For this review, take the finished solid that the model builds, in its own axes (mm). A direction names the side the tool comes from. Round coordinates to 2 decimals unless told otherwise and drop trailing zeros. Order: outer loops, then holes, each group sorted by start corner. A loop starts at its lowest first (then second) coordinate and runs counter-clockwise, first axis right, second up. Notation, with made-up numbers: (24.25, -22) - (54.25, -22) arc R17 cw to (54.25, -14) - close; hole circle Ø5 at (35, 89). An arc over 180 degrees is marked (long way). Write each question's results on one line, items separated by ' | '. Start each with the question number.
(1) Take a section at C-C, the plane y = 1. Give the boundary of the cut face in (x, z).
(2) Insertion check: pin 1 Ø4 at (x, z) = (10, 32.5) entering from -Y; pin 2 Ø3 at (x, y) = (14.5, 9) entering from +Z. Each pin has a flat end and moves straight along its axis. Give the tip position at first contact, or say it passes through.
(3) Take a section at A-A, the plane y = 8.75. Give the boundary of the cut face in (x, z).
(4) For faces 1 (the flat face through (0, 9, 24)), 2 (the cylindrical face through (8.19, 7.4, 50.96)), list the 3-axis set-ups (+Z, -Z, +X, -X, +Y, -Y) from which the entire face can be reached by the end or side of a thin tool; tool diameter is ignored.
(5) For L1, parallel to Z at x = 17.5, y = 6, list the stretches that pass through material, from the lowest coordinate up. Write a range as from..to.
(6) Take a section at B-B, the plane x = 13. Give the boundary of the cut face in (y, z).
(7) Draft analysis for pull direction Y (two halves, no side actions). For faces 3 (the flat face through (26.5, 9, 24)), 4 (the flat face through (7, 9, 48.5)), 5 (the cylindrical face through (18.01, 8.15, 50.96)), state which applies: pulls with the +Y half, pulls with the -Y half, needs draft (parallel to the pull), parting line crosses it, or undercut.
```python
from build123d import *

# Parameters (mm, degrees)
SKETCH1_W           = 26.5
SKETCH1_H           = 17.5
BOSS_EXTRUDE1_DEPTH = 48.5
SKETCH2_R           = 2
SKETCH2_R_2         = 1
SKETCH2_R_3         = 4
BOSS_EXTRUDE2_DEPTH = 5


with BuildPart() as part:
    # Sketch1 → Boss-Extrude1 (new body)
    with BuildSketch(Plane.XY):
        with Locations((13.25, 8.75)):
            Rectangle(SKETCH1_W, SKETCH1_H)
    extrude(amount=BOSS_EXTRUDE1_DEPTH)

    # Sketch2 → Boss-Extrude2 (add)
    # profile 1 of 2: a face of its own
    with BuildSketch(Plane.XY.offset(48.5)):
        with Locations(Location((19.919028118, 8.75, 0), (0, 0, 180))):
            Circle(SKETCH2_R)
        with Locations((19.919028118, 8.75)):
            Circle(SKETCH2_R_2, mode=Mode.SUBTRACT)
    # profile 2 of 2: a face of its own
    with BuildSketch(Plane.XY.offset(48.5)):
        with Locations(Location((6.714907482, 8.75, 0), (0, 0, 180))):
            Circle(SKETCH2_R_3)
        with Locations(Location((6.714907482, 8.75, 0), (0, 0, 180))):
            Circle(SKETCH2_R, mode=Mode.SUBTRACT)
    extrude(amount=BOSS_EXTRUDE2_DEPTH)


solid = part.part
```
Results below:
1) outline: (0, 0) - (26.5, 0) - (26.5, 48.5) - (0, 48.5) - close
2) pin 1: stops at y = 0 | pin 2: stops at z = 48.5
3) outline: (0, 0) - (26.5, 0) - (26.5, 48.5) - (21.92, 48.5) - (21.92, 53.5) - (20.92, 53.5) - (20.92, 48.5) - (18.92, 48.5) - (18.92, 53.5) - (17.92, 53.5) - (17.92, 48.5) - (10.71, 48.5) - (10.71, 53.5) - (8.71, 53.5) - (8.71, 48.5) - (4.71, 48.5) - (4.71, 53.5) - (2.71, 53.5) - (2.71, 48.5) - (0, 48.5) - close
4) face 1: +Z, -Z, -X, +Y, -Y | face 2: +Z
5) L1: z = 0..48.5
6) outline: (0, 0) - (17.5, 0) - (17.5, 48.5) - (0, 48.5) - close
7) face 3: needs draft | face 4: undercut | face 5: parting line crosses it
